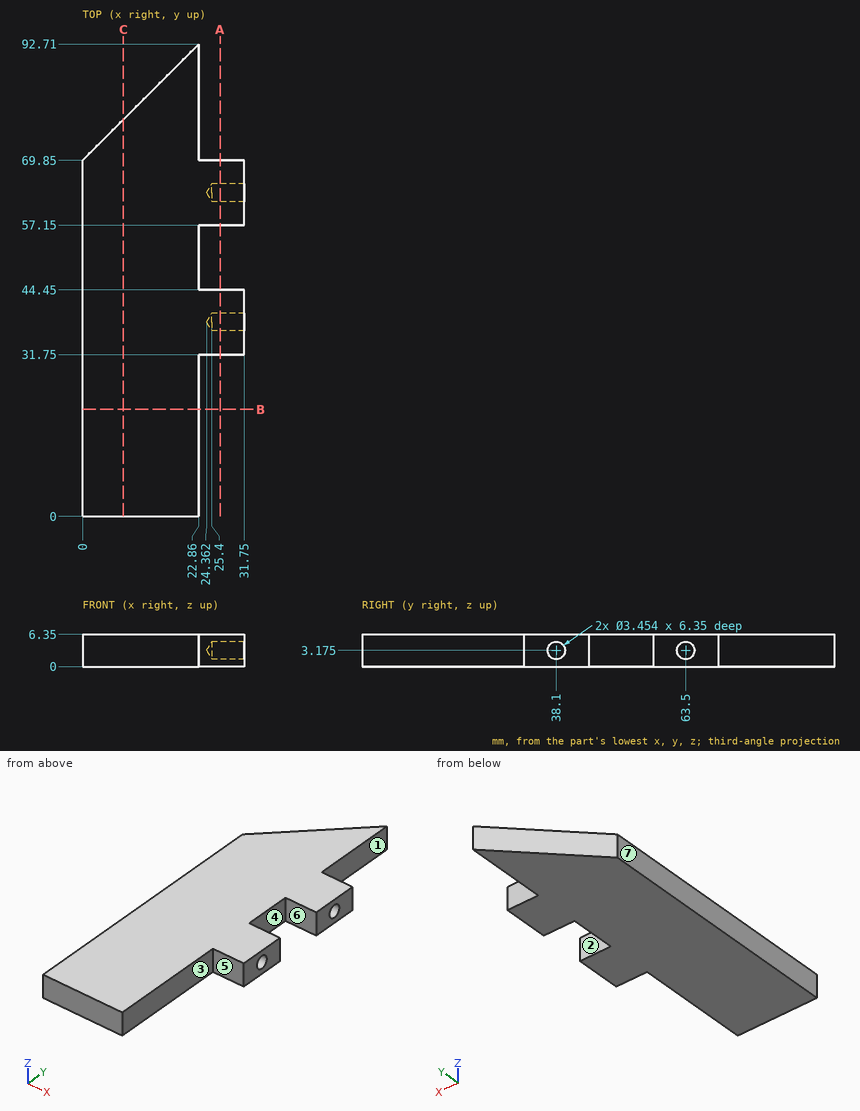
Can you work these out from the drawing? Everything is in mm from the part's minimum corner. A direction names the side the tool comes from. Give positions to 0.01 mm unless a question says otherwise; leave off trailing zeros. Loops run counter-clockwise (first coordinate to the right, second up) from the corner with the lowest first, then second, coordinate; pieces in that order, holes last. Notation, with made-up numbers: (50.5, -27) -> (55.5, -27) arc R15 cw to (55.5, -22) -> close; hole circle Ø5 at (82.25, 3.25). An arc over 180 degrees is marked (long way). Return JSON: item names as keys, results as strings.
Item 1: If we section it at B-B on y = 21: List the corners of the cut face in (x, z) for me, plus the area to 3 significant figures.
Geometry results:
{"outline": "(0, 0) -> (22.86, 0) -> (22.86, 6.35) -> (0, 6.35) -> close", "area": "145 mm²"}
Item 2: I need wall thicknesses on L1, parallel to Z at x = 29.25, y = 38.1; L2, parallel to Y at x = 24, z = 4; L3, parallel to Y at x = 27, z = 2.25. Which ranges of each line are inside material? Lowest first, please. Write a range as from..to.
Geometry results:
{"L1": "z = 0..1.45, 4.9..6.35", "L2": "y = 31.75..44.45, 57.15..69.85", "L3": "y = 31.75..36.64, 39.56..44.45, 57.15..62.04, 64.96..69.85"}
Item 3: Which directions (+Z, -Z, +X, -X, +Y, -Y) give clear straight access to the entire face, cutting with the end or side of a thin tool? Please do the marked faces 1, 2 and 3.
Geometry results:
{"face 1": "+Z, -Z, +X, +Y", "face 2": "+Z, -Z, +X", "face 3": "+Z, -Z, +X, -Y"}
Item 4: I'm going to push flat-ended pins straight in: pin 1 (3 mm diameter, centred on y = 85.5, z = 2.5, fed in from +X); pin 2 (1.9 mm diameter, centred on x = 25.5, z = 2.5, fed in from -Y); pin 3 (1.9 mm diameter, centred on x = 27.5, z = 2.5, fed in from +Y). Where does each tip first touch, or does it pass through?
Geometry results:
{"pin 1": "stops at x = 22.86", "pin 2": "stops at y = 31.75", "pin 3": "stops at y = 69.85"}
Item 5: If we section it at C-C on x = 8: List the corners of the cut face in (y, z) for me, plus the area to 3 significant figures.
Geometry results:
{"outline": "(0, 0) -> (77.85, 0) -> (77.85, 6.35) -> (0, 6.35) -> close", "area": "494 mm²"}
Item 6: If we section it at A-A on x = 27: Count the separate pieces of the cut face and the enclosed holes in it.
Geometry results:
{"separate pieces": "2", "enclosed holes": "2"}
Item 7: We'd pull the mould along Y, two halves only. Please class the marked faces 4, 5, 6 and 7: +Y half, -Y half, draft (parallel to the pull), parting line (faces both ways), or undercut.
Geometry results:
{"face 4": "undercut", "face 5": "-Y half", "face 6": "undercut", "face 7": "draft"}
